Autodesk Inventor part; units mm, degrees
ref_plane "YZ Plane" through (0, 0, 0) normal (1, 0, 0) x (0, 1, 0)
ref_plane "XZ Plane" through (0, 0, 0) normal (0, 1, 0) x (-1, 0, 0)
ref_plane "XY Plane" through (0, 0, 0) normal (0, 0, 1) x (1, 0, 0)
sketch "Sketch1" plane through (0, 0, 0) normal (0, 0, 1) x (1, 0, 0)
  line L0 (0, 0) -> (50, 0)
  line L1 (50, 0) -> (50, 10.3348)
  line L2 (0, 0) -> (0, 19) construction
  arc A0 (0, 8) -> (6.6332, 19) centre (0, 15.5) ccw
  line L3 (6.6332, 19) -> (11.8173, 19)
  line L4 (48.3623, 12.3017) -> (12.1797, 18.9669)
  arc A1 (12.1797, 18.9669) -> (11.8173, 19) centre (11.8173, 17) ccw
  arc A2 (50, 10.3348) -> (48.3623, 12.3017) centre (48, 10.3348) ccw
  line L5 (0, 0) -> (0, 8)
  point P0 (50, 12)
  point P1 (12, 19)
  dimension "d0" = 50
  dimension "d1" = 12
  dimension "d2" = 19
  dimension "d3" = 15
  dimension "d4" = 3.5
  dimension "d5" = 12
  dimension "d6" = 2
  dimension "d14" = 19
revolve "Revolution1" add sketch "Sketch1" angle 360 about axis through (0, 0, 0) along (0, 1, 0)
sketch "Sketch2" plane through (0, 0, 0) normal (0, -1, 0) x (1, 0, 0)
  circle A0 centre (0, 0) radius 50
  circle A1 centre (0, 0) radius 7.5
  dimension "d8" = 15
extrude "Extrusion1" cut sketch "Sketch2" against normal blind 1 contours A1
sketch "Sketch3" plane through (0, 0, 0) normal (0, -1, 0) x (1, 0, 0)
  circle A0 centre (0, 0) radius 7.5
  circle A1 centre (0, 0) radius 50
  circle A2 centre (0, 0) radius 46
  dimension "d11" = 4
extrude "Extrusion2" cut sketch "Sketch3" against normal blind 5 contours A2
sketch "Sketch4" plane through (0, 5, 0) normal (0, -1, 0) x (1, 0, 0)
  circle A0 centre (0, 0) radius 7.5
  arc A1 (-37, 10) -> (-37, -10) centre (-37, 0) ccw
  arc A2 (37, -10) -> (37, 10) centre (37, 0) ccw
  line L0 (12, 10) -> (12, -10)
  line L1 (-12, 10) -> (-12, -10)
  line L2 (-37, 10) -> (-12, 10)
  line L3 (-37, -10) -> (-12, -10)
  line L4 (12, 10) -> (37, 10)
  line L5 (12, -10) -> (37, -10)
  point P0 (-12, 0)
  point P1 (12, 0)
  dimension "d15" = 20
  dimension "d16" = 20
  dimension "d17" = 74
  dimension "d18" = 37
  dimension "d19" = 20
  dimension "d20" = 20
  dimension "d21" = 25
  dimension "d22" = 25
extrude "Extrusion3" add sketch "Sketch4" against normal blind 13 contours L2 L1 L3 A1 | L5 L0 L4 A2
fillet "Fillet1" radius 2 6 edges at (-25.6371, 18, 10) (-47, 18, 0) (-25.6371, 18, -10) (25.6371, 18, 10) (47, 18, 0) (25.6371, 18, -10)
sketch "Sketch5" plane through (0, 5, 0) normal (0, -1, 0) x (1, 0, 0)
  arc A0 (-37, 10) -> (-37, -10) centre (-37, 0) ccw
  circle A1 centre (-37, 0) radius 4.5
  circle A2 centre (37, 0) radius 4.5
  dimension "d26" = 9
  dimension "d27" = 9
extrude "Extrusion4" cut sketch "Sketch5" against normal through all
equation "\"d18\" = 0.5 * d17"
equation "\"d22\" = d21"
equation "\"d27\" = d26"
properties part number "PAD 100mm GRAY PLASTIC WITH ATTACHMENT BORES" material "ABS Plastic"
Check sheet for the modelled part. Datum: model origin and axes. Units: mm. A direction names the side the tool comes from. Coordinates: 2 decimals unless noted, no trailing zeros. Write each loop counter-clockwise with the first axis right and the second up, starting at its lowest first coordinate (ties: lowest second). Pieces come first, ordered by that corner, then holes.
Item 1: Cross-section at A-A on y = 6.25. Record the boundary of the cut face in (x, z), then the cut area to 3 significant figures.
Numbers:
outline: circle Ø100 at (0, 0); hole circle Ø9 at (-37, 0); hole circle Ø9 at (37, 0)
area: 7,730 mm2
Item 2: Depth check by flat-ended pin: pin 1 Ø2 at (x, z) = (11, 35.5) entering from -Y; pin 2 Ø3 at (x, z) = (-30.5, -38.5) entering from +Y; pin 3 Ø4.5 at (x, z) = (0, 1.5) entering from -Y; pin 4 Ø5.5 at (x, z) = (37, 0) entering from +Y. Enter the tip coordinate at first touch or a pass-through.
Numbers:
pin 1: stops at y = 5
pin 2: stops at y = 12.44
pin 3: stops at y = 1
pin 4: passes through
Item 3: Access from +Z, -Z, +X, -X, +Y, -Y to the whole of each face (thin tool, end or side, straight path). Record for faces 1 (the face through (41.292, 11.409, 1.352)), 2 (the face through (47, 15, 0)), 3 (the face through (-5.99, 2.46, 45.61)), 4 (the face through (-47, 15, 0)).
Numbers:
face 1: +Y, -Y
face 2: +X, +Y
face 3: -Y
face 4: -X, +Y
Item 4: Scan lines: probe 1 along Z at (x, y) = (0, 3.5); probe 2 along Y at (x, z) = (34.5, 34); probe 3 along Y at (x, z) = (28.5, -7.5). Record each from-to range of solid material in increasing order.
Numbers:
probe 1: z = -50 to -46, -7.5 to 7.5, 46 to 50
probe 2: y = 0 to 12.29
probe 3: y = 5 to 18
